Check sheet for the modelled part. Datum: model origin and axes. Units: mm. A direction names the side the tool comes from. Coordinates: 2 decimals unless noted, no trailing zeros. Loops run counter-clockwise (first coordinate to the right, second up) from the corner with the lowest first, then second, coordinate; pieces in that order, holes last.
Autodesk Inventor part; units mm, degrees
ref_plane "YZ Plane" through (0, 0, 0) normal (1, 0, 0) x (0, 1, 0)
ref_plane "XZ Plane" through (0, 0, 0) normal (0, 1, 0) x (-1, 0, 0)
ref_plane "XY Plane" through (0, 0, 0) normal (0, 0, 1) x (1, 0, 0)
sketch "Sketch1" plane through (0, 0, 0) normal (0, 0, 1) x (1, 0, 0)
  line L0 (0, 0) -> (12.5, 0)
  line L1 (12.5, 0) -> (12.5, 5)
  line L2 (12.5, 5) -> (0, 5)
  line L3 (0, 5) -> (0, 0)
  line L4 (0, 0) -> (5, 0) construction
  line L5 (12.5, 0) -> (7.5, 0) construction
  line L6 (0, 0) -> (5, 0) construction
  line L7 (5, 0) -> (5, -49.5) construction
  line L8 (5, -49.5) -> (0, -49.5) construction
  line L9 (0, -49.5) -> (0, 0) construction
  line L10 (0, 0) -> (5, 0)
  line L11 (5, 0) -> (5, -49.5)
  line L12 (5, -49.5) -> (0, -49.5)
  line L13 (0, -49.5) -> (0, 0)
  line L14 (7.5, 0) -> (12.5, 0)
  line L15 (12.5, 0) -> (12.5, -49.5)
  line L16 (12.5, -49.5) -> (7.5, -49.5)
  line L17 (7.5, -49.5) -> (7.5, 0)
  dimension "d0" = 12.5
  dimension "d1" = 5
  dimension "d2" = 5
  dimension "d3" = 5
  dimension "d4" = 49.5
extrude "Extrusion1" add sketch "Sketch1" along normal blind 5 contours L0 L11 L12 L13 | L0 L15 L16 L17
sketch "Sketch2" plane through (0, 0, 0) normal (0, 0, -1) x (-1, 0, 0)
  line L0 (-12.5, -49.5) -> (-12.5, 0)
  line L1 (-7.5, -49.5) -> (-12.5, -49.5)
  line L2 (-7.5, 0) -> (-7.5, -49.5)
  line L3 (-12.5, 0) -> (-7.5, 0)
  line L4 (0, -49.5) -> (-5, -49.5)
  line L5 (0, 0) -> (0, -49.5)
  line L6 (-5, 0) -> (0, 0)
  line L7 (-5, -49.5) -> (-5, 0)
  line L8 (-12.5, 0) -> (0, 0)
  line L9 (0, 0) -> (0, 3.75)
  line L10 (0, 3.75) -> (-12.5, 3.75)
  line L11 (-12.5, 3.75) -> (-12.5, 0)
  line L12 (0, -49.5) -> (-5, -49.5)
  line L13 (0, -49.5) -> (-12.5, -49.5)
  line L14 (-12.5, -49.5) -> (-12.5, -53.25)
  line L15 (-12.5, -53.25) -> (0, -53.25)
  line L16 (0, -53.25) -> (0, -49.5)
  point P0 (-5, -49.5)
  point P1 (-7.5, -49.5)
  dimension "d7" = 3.75
  dimension "d10" = 3.75
extrude "Extrusion2" add sketch "Sketch2" against normal blind 15 contours L1 L13 L4 L16 L15 L14 | L11 L10 L9 L6 L8 L3
sketch "Sketch4" plane through (0, -53.25, 0) normal (0, -1, 0) x (1, 0, 0)
  line L0 (7.5, 5) -> (12.5, 5)
  line L1 (0, 5) -> (5, 5)
  line L2 (12.5, 5) -> (12.5, 15) construction
  line L3 (12.5, 0) -> (0, 0) construction
  line L4 (12.5, 15) -> (0, 15) construction
  line L5 (0, 15) -> (0, 0) construction
  line L6 (0, 0) -> (12.5, 0) construction
  line L7 (12.5, 0) -> (12.5, 15) construction
  line L8 (12.5, 15) -> (0, 15) construction
  line L9 (0, 5) -> (12.5, 5) construction
  line L10 (12.5, 5) -> (12.5, 15) construction
  line L11 (12.5, 15) -> (0, 15) construction
  line L12 (0, 15) -> (0, 5) construction
  circle A0 centre (6.25, 10) radius 1.5
  dimension "d12" = 3
extrude "Extrusion3" cut sketch "Sketch4" against normal blind 10
sketch "Sketch5" plane through (0, 3.75, 0) normal (0, 1, 0) x (1, 0, 0)
  line L0 (5, -5) -> (0, -5)
  line L1 (12.5, -5) -> (7.5, -5)
  line L2 (0, 0) -> (12.5, 0)
  line L3 (0, 0) -> (0, -15)
  line L4 (12.5, -15) -> (0, -15)
  line L5 (12.5, 0) -> (12.5, -15)
  line L6 (0, 0) -> (0, -15) construction
  line L7 (7.5, -5) -> (12.5, -5) construction
  line L8 (0, 0) -> (12.5, 0) construction
  line L9 (12.5, 0) -> (12.5, -5) construction
  line L10 (12.5, -5) -> (0, -5) construction
  line L11 (0, -5) -> (0, 0) construction
  line L12 (12.5, 0) -> (12.5, -15)
  line L13 (12.5, -15) -> (0, -15)
  line L14 (0, -15) -> (0, -10)
  line L15 (0, -10) -> (12.5, -10)
  line L16 (12.5, -10) -> (12.5, -15)
  point P0 (0, -10)
  dimension "d15" = 12.5
  dimension "d16" = 15
  dimension "d17" = 5
  dimension "d18" = 5
extrude "Extrusion4" add sketch "Sketch5" along normal blind 10 contours L15 L5 L4 L3
sketch "Sketch6" plane through (0, 0, 15) normal (0, 0, 1) x (1, 0, 0)
  line L0 (0, 3.75) -> (12.5, 3.75)
  line L1 (0, 13.75) -> (12.5, 13.75)
  line L2 (0, 0) -> (0, 13.75) construction
  line L3 (0, 3.75) -> (12.5, 3.75) construction
  line L4 (0, 13.75) -> (12.5, 13.75) construction
  line L5 (12.5, 13.75) -> (12.5, 3.75) construction
  line L6 (12.5, 3.75) -> (0, 3.75) construction
  line L7 (0, 3.75) -> (0, 13.75) construction
  circle A0 centre (6.25, 8.75) radius 1.5
  dimension "d21" = 3
extrude "Extrusion5" cut sketch "Sketch6" against normal blind 10
properties part number "PistaSistBloq"
(1) Section check D-D, the plane x = 2.5. Enter the section's corners in (y, z).
(2) Section check B-B, the plane y = 8.75. Enter the section's corners in (x, z).
(3) Set-up check for faces 5 (the face through (12.5, -20, 4)), 6 (the face through (5.06, -51.4, 9.09)), 7 (the face through (6, -51, 15)), 8 (the face through (10, -24, 5)), 9 (the face through (5, -24, 2)): record each of +Z, -Z, +X, -X, +Y, -Y from which the full face is reachable in a straight line by a thin tool's end or side.
(4) Gauge pin test, flat ends, axial feed: P1, Ø2.5, axis at x = 3, y = -28.5, coming from the +Z side; P2, Ø4, axis at x = 10.5, z = 5.5, coming from the +Y side; P3, Ø4, axis at x = 6.25, y = 8.75, coming from the -Z side. Record the tip position at first contact, or that the pin passes through.
(5) Scan lines: line 1 along Y through (x, z) = (6.25, 12.8); line 2 along Y through (x, z) = (10.25, 13.25); line 3 along X through (y, z) = (-38, 3.5). Record each from-to range of solid material in increasing order.
(6) Section check C-C, the plane x = 6.25. Enter the section's corners in (y, z).
(7) Draft check along Y on faces 1 (the face through (5, 10, 10)), 2 (the face through (7.5, -25, 2)), 3 (the face through (6, -53.25, 7)), 4 (the face through (6, 3.75, 5)). Enter one of: pulls with the +Y half, pulls with the -Y half, needs draft (parallel to the pull), parting line crosses it, or undercut.
(8) Section check A-A, the plane z = 6. Enter the section's corners in (x, y), plus the area to 4 significant figures.
Determined:
1. outline: (-53.25, 0) - (3.75, 0) - (3.75, 10) - (13.75, 10) - (13.75, 15) - (0, 15) - (0, 5) - (-49.5, 5) - (-49.5, 15) - (-53.25, 15) - close
2. outline: (0, 10) - (4.75, 10) - (4.75, 15) - (0, 15) - close; (7.75, 10) - (12.5, 10) - (12.5, 15) - (7.75, 15) - close
3. face 5: +Z, -Z, +X, +Y, -Y
3. face 6: -Y
3. face 7: +Z, +X, -X, +Y, -Y
3. face 8: +Z, +X, -X
3. face 9: +Z, -Z
4. P1: stops at z = 5
4. P2: stops at y = 3.75
4. P3: stops at z = 10
5. line 1: y = -53.25 to -49.5, 0 to 7.25, 10.25 to 13.75
5. line 2: y = -53.25 to -49.5, 0 to 13.75
5. line 3: x = 0 to 5, 7.5 to 12.5
6. outline: (-53.25, 0) - (-49.5, 0) - (-49.5, 8.5) - (-53.25, 8.5) - close; (-53.25, 11.5) - (-49.5, 11.5) - (-49.5, 15) - (-53.25, 15) - close; (0, 0) - (3.75, 0) - (3.75, 10) - (7.25, 10) - (7.25, 15) - (0, 15) - close; (10.25, 10) - (13.75, 10) - (13.75, 15) - (10.25, 15) - close
7. face 1: needs draft
7. face 2: undercut
7. face 3: pulls with the -Y half
7. face 4: pulls with the +Y half
8. outline: (0, -53.25) - (12.5, -53.25) - (12.5, -49.5) - (0, -49.5) - close; (0, 0) - (12.5, 0) - (12.5, 3.75) - (0, 3.75) - close
8. area: 93.75 mm2
